Check sheet for the modelled part. Datum: model origin and axes. Units: mm. A direction names the side the tool comes from. Round coordinates to 2 decimals unless told otherwise and drop trailing zeros. Order: outer loops, then holes, each group sorted by start corner. A loop starts at its lowest first (then second) coordinate and runs counter-clockwise, first axis right, second up. Notation, with made-up numbers: (-2, -21.5) -> (29, -21.5) arc R23 ccw to (29, 3.5) -> close; hole circle Ø6 at (41.5, -30.75). An arc over 180 degrees is marked (long way). Answer in a Markdown table with one row per item.
Autodesk Inventor part; units mm, degrees
ref_plane "YZ Plane" through (0, 0, 0) normal (1, 0, 0) x (0, 1, 0)
ref_plane "XZ Plane" through (0, 0, 0) normal (0, 1, 0) x (-1, 0, 0)
ref_plane "XY Plane" through (0, 0, 0) normal (0, 0, 1) x (1, 0, 0)
sketch "Esquisse1" plane through (0, 0, 0) normal (0, 1, 0) x (-1, 0, 0)
  line L0 (15, 25) -> (-15, 25)
  line L1 (-15, 25) -> (-15, -25)
  line L2 (-15, -25) -> (15, -25)
  line L3 (15, -25) -> (15, 25)
  line L4 (15, 25) -> (-15, -25)
  line L5 (-15, 25) -> (15, -25)
  circle A0 centre (0, 14) radius 4.05
  line L6 (21, 0) -> (-18, 0)
  circle A1 centre (0, -14) radius 4.05
  point P0 (0, 0)
  point P1 (0, 0)
  point P2 (0, 0)
  dimension "d0" = 50
  dimension "d1" = 30
  dimension "d2" = 8.1
  dimension "d3" = 14
extrude "Extrusion1" add sketch "Esquisse1" along normal blind 10 contours L4 L5 L0 | L3 L6 L4 | L5 L6 L1 | L3 L5 L6 | L5 L2 L4 | L4 L1 L6 | A0 | A1
sketch "Esquisse2" plane through (0, 10, 0) normal (0, 1, 0) x (1, 0, 0)
  circle A0 centre (0, -13) radius 4.05
  line L0 (-17, 0) -> (22, 0)
  circle A1 centre (0, 13) radius 4.05
  line L1 (-15, 25) -> (-15, -25)
  line L2 (15, -25) -> (15, 25)
  line L3 (-15, -25) -> (15, -25)
  line L4 (15, -25) -> (15, 25)
  line L5 (15, 25) -> (-15, 25)
  line L6 (-15, 25) -> (-15, -25)
  point P0 (0, 0)
  dimension "d6" = 8.1
  dimension "d7" = 13
extrude "Extrusion2" add sketch "Esquisse2" along normal blind 15
sketch "Esquisse3" plane through (0, 0, 0) normal (0, -1, 0) x (1, 0, 0)
  line L0 (-15, -25) -> (-15, 25)
  line L1 (15, 25) -> (15, -25)
  line L2 (-15, -8.05) -> (15, -8.05)
  line L3 (15, -8.05) -> (15, 8.05)
  line L4 (15, 8.05) -> (-15, 8.05)
  line L5 (-15, 8.05) -> (-15, -8.05)
  line L6 (-15, -8.05) -> (15, 8.05)
  line L7 (15, -8.05) -> (-15, 8.05)
  line L8 (15, -25) -> (-15, -25)
  line L9 (-15, 25) -> (15, 25)
  line L10 (-15, -25) -> (15, -25)
  line L11 (15, -25) -> (15, 25)
  line L12 (15, 25) -> (-15, 25)
  line L13 (-15, 25) -> (-15, -25)
  point P0 (0, 0)
  point P1 (0, 0)
  point P2 (0, 0)
  point P3 (-15, 8.05)
  point P4 (15, -8.05)
  dimension "d10" = 16.1
extrude "Extrusion3" add sketch "Esquisse3" along normal blind 17 contours L0 L2 L1 L8 | L0 L9 L1 L4
sketch "Esquisse4" plane through (-15, 25, 25) normal (0, 0, 1) x (1, 0, 0)
  line L0 (30, -25) -> (30, -42)
  line L1 (30, -25) -> (0, -25)
  line L2 (30, -42) -> (0, -42)
  line L3 (0, -42) -> (0, -25)
  line L4 (0, -25) -> (30, -25)
  line L5 (30, -25) -> (30, -42)
  circle A0 centre (15, -33.5) radius 2.9
  point P0 (15, -25)
  dimension "d13" = 5.8
extrude "Extrusion4" cut sketch "Esquisse4" against normal blind 50 contours A0
sketch "Esquisse5" plane through (0, 0, 0) normal (0, -1, 0) x (1, 0, 0)
  line L0 (15, -8.05) -> (-15, -8.05)
  line L1 (-15, 8.05) -> (15, 8.05)
  line L2 (-8, -8.05) -> (8, -8.05)
  line L3 (8, -8.05) -> (8, 8.05)
  line L4 (8, 8.05) -> (-8, 8.05)
  line L5 (-8, 8.05) -> (-8, -8.05)
  line L6 (-8, -8.05) -> (8, 8.05)
  line L7 (8, -8.05) -> (-8, 8.05)
  line L8 (-15, -8.05) -> (15, -8.05)
  line L9 (15, -8.05) -> (15, 8.05)
  line L10 (15, 8.05) -> (-15, 8.05)
  line L11 (-15, 8.05) -> (-15, -8.05)
  point P0 (0, 0)
  point P1 (0, 0)
  point P2 (0, 0)
  point P3 (8, -8.05)
  point P4 (-8, 8.05)
  dimension "d16" = 16
extrude "Extrusion5" cut sketch "Esquisse5" against normal blind 25 contours L0 L3 L1 L9 | L0 L11 L1 L5
(1) Scan lines: probe 1 along Z at (x, y) = (0, 13.25); probe 2 along Z at (x, y) = (-11, -1); probe 3 along X at (y, z) = (20, -13). Record each from-to range of solid material in increasing order. Write a range as from..to.
Solutions:
| item | result |
|---|---|
| probe 1 | -25..-17.05, -8.95..8.95, 17.05..25 |
| probe 2 | -25..-8.05, 8.05..25 |
| probe 3 | -15..-4.05, 4.05..15 |
(2) Section check A-A on x = 0. Record the boundary of the cut face in (y, z), plus the area to 3 significant figures.
Solutions:
| item | result |
|---|---|
| outline | (-17, -25) -> (-11.4, -25) -> (-11.4, -8.05) -> (-17, -8.05) -> close; (-17, 8.05) -> (-11.4, 8.05) -> (-11.4, 25) -> (-17, 25) -> close; (-5.6, -25) -> (25, -25) -> (25, -17.05) -> (10, -17.05) -> (10, -8.95) -> (25, -8.95) -> (25, 8.95) -> (10, 8.95) -> (10, 17.05) -> (25, 17.05) -> (25, 25) -> (-5.6, 25) -> (-5.6, 8.05) -> (0, 8.05) -> (0, -8.05) -> (-5.6, -8.05) -> close |
| area | 1,390 mm^2 |
(3) Section check D-D on z = -13. Record the boundary of the cut face in (x, y).
Solutions:
| item | result |
|---|---|
| outline | (-15, -17) -> (15, -17) -> (15, 25) -> (4.05, 25) -> (4.05, 10) -> (-4.05, 10) -> (-4.05, 25) -> (-15, 25) -> close; hole circle Ø5.8 at (0, -8.5) |
(4) Section check C-C on x = -12. Record the boundary of the cut face in (y, z), plus the area to 3 significant figures.
Solutions:
| item | result |
|---|---|
| outline | (-17, -25) -> (25, -25) -> (25, -8.05) -> (-17, -8.05) -> close; (-17, 8.05) -> (25, 8.05) -> (25, 25) -> (-17, 25) -> close |
| area | 1,420 mm^2 |
(5) Tool access check on faces 1 (the flat face through (0.2, -0.4, 8.05)), 2 (the flat face through (-8, 12, 0)), 3 (the cylindrical face through (-0.878, 17.395, 9.046)). Record the directions out of +Z, -Z, +X, -X, +Y, -Y that give a thin tool (end or side, any length) a straight path to the whole face; none if there is none.
Solutions:
| item | result |
|---|---|
| face 1 | -Y |
| face 2 | -X, +Y, -Y |
| face 3 | +Y |
(6) Depth check by flat-ended pin: pin 1 Ø6 at (y, z) = (-12.5, 4.5) entering from -X (3 decimals); pin 2 Ø5 at (y, z) = (12, -2) entering from +X; pin 3 Ø17.5 at (y, z) = (17, -0.5) entering from -X; pin 4 Ø2.5 at (x, z) = (-1, -13) entering from +Y. Enter the tip coordinate at first touch or a pass-through.
Solutions:
| item | result |
|---|---|
| pin 1 | through |
| pin 2 | x = 8 |
| pin 3 | x = -15 |
| pin 4 | y = 10 |
(7) Section check B-B on y = -8.5. Record the boundary of the cut face in (x, z), plus the area to 3 significant figures.
Solutions:
| item | result |
|---|---|
| outline | (-15, -25) -> (-2.9, -25) -> (-2.9, -8.05) -> (-15, -8.05) -> close; (-15, 8.05) -> (-2.9, 8.05) -> (-2.9, 25) -> (-15, 25) -> close; (2.9, -25) -> (15, -25) -> (15, -8.05) -> (2.9, -8.05) -> close; (2.9, 8.05) -> (15, 8.05) -> (15, 25) -> (2.9, 25) -> close |
| area | 820 mm^2 |
(8) Draft check along Z on faces 4 (the flat face through (0, 10, 13)), 5 (the flat face through (0, 4, -25)), 6 (the flat face through (0, -1, -8.05)), 7 (the flat face through (0, -17, -16)). Enter one of: pulls with the +Z half, pulls with the -Z half, needs draft (parallel to the pull), parting line crosses it, or undercut.
Solutions:
| item | result |
|---|---|
| face 4 | undercut |
| face 5 | pulls with the -Z half |
| face 6 | undercut |
| face 7 | needs draft |
